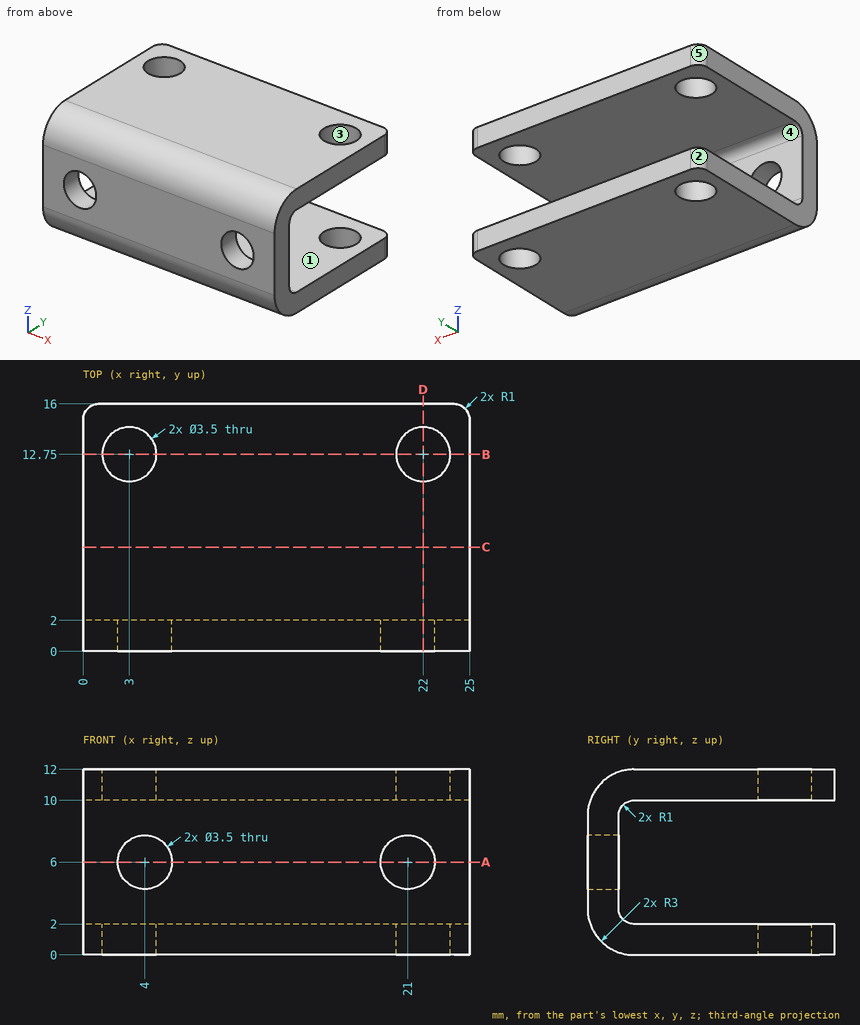
Here's the drawing with two shaded views (mm, measured from the low corner). I have some questions. A direction names the side the tool comes from. Round coordinates to 2 decimals unless told otherwise and drop trailing zeros. Write each loop counter-clockwise with the first axis right and the second up, starting at its lowest first coordinate (ties: lowest second). Pieces come first, ordered by that corner, then holes. Notation, with made-up numbers: M 22,50 L 80,50 A19 cw 80,83 Z; hole C 88,-23 d11. An arc over 180 degrees is marked long. Use CSV: the item, a comma, the result in double quotes.
(1) Imagine slicing it at A-A (z = 6). Write out the boundary of the cut face in (x, y).
Check values:
outline,"M 0,0 L 2.25,0 L 2.25,2 L 0,2 Z; M 5.75,0 L 19.25,0 L 19.25,2 L 5.75,2 Z; M 22.75,0 L 25,0 L 25,2 L 22.75,2 Z"
(2) I'm going to push flat-ended pins straight in: pin 1 (4 mm diameter, centred on x = 21, z = 6, fed in from +Y); pin 2 (2 mm diameter, centred on y = 2.5, z = 9.5, fed in from -X). Where does each tip first touch, or does it pass through?
Check values:
pin 1,"y = 2"
pin 2,"x = 0"
(3) Imagine slicing it at D-D (x = 22). Write out the boundary of the cut face in (y, z).
Check values:
outline,"M 0,3 A3 ccw 3,0 L 11,0 L 11,2 L 3,2 A1 cw 2,3 L 2,4.56 L 0,4.56 Z; M 0,7.44 L 2,7.44 L 2,9 A1 cw 3,10 L 11,10 L 11,12 L 3,12 A3 ccw 0,9 Z; M 14.5,0 L 16,0 L 16,2 L 14.5,2 Z; M 14.5,10 L 16,10 L 16,12 L 14.5,12 Z"
(4) On a 3-axis mill with a long thin cutter (end or side, diameter ignored), from which of +Z, -Z, +X, -X, +Y, -Y can I reach the whole of each face in a straight line? I mean the marked faces 4 and 5. Say none if no direction works.
Check values:
face 4,"+X, -X, +Y"
face 5,"+Z, -Z, -X, +Y"
(5) Imagine slicing it at B-B (y = 12.75). Write out the boundary of the cut face in (x, z).
Check values:
outline,"M 0,0 L 1.25,0 L 1.25,2 L 0,2 Z; M 0,10 L 1.25,10 L 1.25,12 L 0,12 Z; M 4.75,0 L 20.25,0 L 20.25,2 L 4.75,2 Z; M 4.75,10 L 20.25,10 L 20.25,12 L 4.75,12 Z; M 23.75,0 L 25,0 L 25,2 L 23.75,2 Z; M 23.75,10 L 25,10 L 25,12 L 23.75,12 Z"
(6) I need wall thicknesses on line 1 along Z through (x, y) = (10.25, 6.25); line 2 along X through (y, z) = (12.75, 11.3); line 3 along Y through (x, z) = (1.5, 3.25). Which ranges of each line are inside material? Lowest first, please.
Check values:
line 1,"0 to 2, 10 to 12"
line 2,"0 to 1.25, 4.75 to 20.25, 23.75 to 25"
line 3,"0 to 2"
(7) We'd pull the mould along Y, two halves only. Please class the marked faces 1, 2 and 3: +Y half, -Y half, draft (parallel to the pull), parting line (faces both ways), or undercut.
Check values:
face 1,"draft"
face 2,"+Y half"
face 3,"undercut"
(8) Imagine slicing it at C-C (y = 6.75). Write out the boundary of the cut face in (x, z), plus the area to 3 significant figures.
Check values:
outline,"M 0,0 L 25,0 L 25,2 L 0,2 Z; M 0,10 L 25,10 L 25,12 L 0,12 Z"
area,"100 mm^2"
